For this review, take the finished solid that the model builds, in its own axes (mm). Face numbers are marked on the shaded views. Coordinates: 2 decimals unless noted, no trailing zeros. Loops run counter-clockwise (first coordinate to the right, second up) from the corner with the lowest first, then second, coordinate; pieces in that order, holes last.
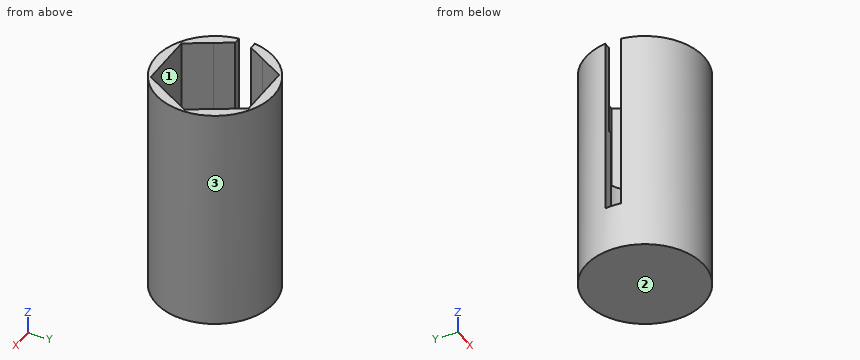
```python
from build123d import *

# Parameters (mm, degrees)
F0_R     = 13
F1_DEPTH = 50
F2_DEPTH = 2
F4_DEPTH = 30
F3_W     = 3.5
F3_H     = 40
F5_DEPTH = 25


with BuildPart() as f1:
    # F0 (on Top) → F1 (new body)
    with BuildSketch(Plane.XY):
        Circle(F0_R)
        Polygon((6.2065153938, 10.75), (9.3097731741, 5.3749998556), (12.4130307876, 0), (9.3097730463, -5.3750000769), (6.2065153938, -10.75), (0, -10.75), (-6.2065153938, -10.75), (-9.3097732188, -5.374999778), (-12.4130307876, 0), (-9.3097730642, 5.3750000458), (-6.2065153938, 10.75), (0, 10.75), align=None, mode=Mode.SUBTRACT)
    extrude(amount=F1_DEPTH)

    # F0 (on Top) → F2 (join)
    with BuildSketch(Plane.XY):
        with BuildLine():
            Line((6.2065153938, -10.75), (9.3097730463, -5.3750000769))
            ThreePointArc((9.3097730463, -5.3750000769), (5.3749999615, -9.3097731129), (0, -10.75))
            Line((0, -10.75), (6.2065153938, -10.75))
        make_face()
        with BuildLine():
            Line((-6.2065153938, -10.75), (0, -10.75))
            ThreePointArc((0, -10.75), (-5.375000111, -9.3097730266), (-9.3097732188, -5.374999778))
            Line((-9.3097732188, -5.374999778), (-6.2065153938, -10.75))
        make_face()
        with BuildLine():
            ThreePointArc((9.3097730463, -5.3750000769), (10.3837026211, -2.7823047777), (10.75, 0))
            ThreePointArc((10.75, 0), (10.3837026542, 2.7823046543), (9.3097731741, 5.3749998556))
            ThreePointArc((9.3097731741, 5.3749998556), (5.3750000722, 9.309773049), (0, 10.75))
            ThreePointArc((0, 10.75), (-5.3749999771, 9.3097731039), (-9.3097730642, 5.3750000458))
            ThreePointArc((-9.3097730642, 5.3750000458), (-10.75, 1.546e-07), (-9.3097732188, -5.374999778))
            ThreePointArc((-9.3097732188, -5.374999778), (-5.375000111, -9.3097730266), (0, -10.75))
            ThreePointArc((0, -10.75), (5.3749999615, -9.3097731129), (9.3097730463, -5.3750000769))
        make_face()
        with BuildLine():
            ThreePointArc((-9.3097730642, 5.3750000458), (-5.3749999771, 9.3097731039), (0, 10.75))
            Line((0, 10.75), (-6.2065153938, 10.75))
            Line((-6.2065153938, 10.75), (-9.3097730642, 5.3750000458))
        make_face()
        with BuildLine():
            ThreePointArc((-9.3097732188, -5.374999778), (-10.75, 1.546e-07), (-9.3097730642, 5.3750000458))
            Line((-9.3097730642, 5.3750000458), (-12.4130307876, 0))
            Line((-12.4130307876, 0), (-9.3097732188, -5.374999778))
        make_face()
        with BuildLine():
            ThreePointArc((0, 10.75), (5.3750000722, 9.309773049), (9.3097731741, 5.3749998556))
            Line((9.3097731741, 5.3749998556), (6.2065153938, 10.75))
            Line((6.2065153938, 10.75), (0, 10.75))
        make_face()
        with BuildLine():
            ThreePointArc((9.3097731741, 5.3749998556), (10.3837026542, 2.7823046543), (10.75, 0))
            ThreePointArc((10.75, 0), (10.3837026211, -2.7823047777), (9.3097730463, -5.3750000769))
            Line((9.3097730463, -5.3750000769), (12.4130307876, 0))
            Line((12.4130307876, 0), (9.3097731741, 5.3749998556))
        make_face()
    extrude(amount=F2_DEPTH)

    # F0 (on Top) → F4 (join)
    with BuildSketch(Plane.XY):
        with BuildLine():
            ThreePointArc((0, 10.75), (5.3750000722, 9.309773049), (9.3097731741, 5.3749998556))
            Line((9.3097731741, 5.3749998556), (6.2065153938, 10.75))
            Line((6.2065153938, 10.75), (0, 10.75))
        make_face()
        with BuildLine():
            ThreePointArc((-9.3097730642, 5.3750000458), (-5.3749999771, 9.3097731039), (0, 10.75))
            Line((0, 10.75), (-6.2065153938, 10.75))
            Line((-6.2065153938, 10.75), (-9.3097730642, 5.3750000458))
        make_face()
        with BuildLine():
            ThreePointArc((-9.3097732188, -5.374999778), (-10.75, 1.546e-07), (-9.3097730642, 5.3750000458))
            Line((-9.3097730642, 5.3750000458), (-12.4130307876, 0))
            Line((-12.4130307876, 0), (-9.3097732188, -5.374999778))
        make_face()
        with BuildLine():
            Line((-6.2065153938, -10.75), (0, -10.75))
            ThreePointArc((0, -10.75), (-5.375000111, -9.3097730266), (-9.3097732188, -5.374999778))
            Line((-9.3097732188, -5.374999778), (-6.2065153938, -10.75))
        make_face()
        with BuildLine():
            Line((6.2065153938, -10.75), (9.3097730463, -5.3750000769))
            ThreePointArc((9.3097730463, -5.3750000769), (5.3749999615, -9.3097731129), (0, -10.75))
            Line((0, -10.75), (6.2065153938, -10.75))
        make_face()
        with BuildLine():
            ThreePointArc((9.3097731741, 5.3749998556), (10.3837026542, 2.7823046543), (10.75, 0))
            ThreePointArc((10.75, 0), (10.3837026211, -2.7823047777), (9.3097730463, -5.3750000769))
            Line((9.3097730463, -5.3750000769), (12.4130307876, 0))
            Line((12.4130307876, 0), (9.3097731741, 5.3749998556))
        make_face()
    extrude(amount=F4_DEPTH)

    # F3 (on Right) → F5 (cut)
    with BuildSketch(Plane.YZ):
        with Locations((0.0118296053, 30.4367649183)):
            Rectangle(F3_W, F3_H)
    extrude(amount=-F5_DEPTH, mode=Mode.SUBTRACT)


solid = f1.part
```
Q1. The part is to be moulded in two halves that separate along Y. For the marked faces 1, 2 and 3, say which applies: +Y half, -Y half, draft (parallel to the pull), parting line (faces both ways), or undercut.
Q2. Consider section A-A (z = 5). State the section outline as (x, y) points, then the cut area to 3 significant figures.
Q3. Consider section D-D (z = 27). State the section outline as (x, y) points.
Q4. Consider section B-B (x = 3.75). State the section outline as (y, z) points.
Q5. Wall thickness on probe 1 along Y at (x, z) = (0, 15); probe 2 along Z at (x, y) = (8, 3.25); probe 3 along X at (y, z) = (0, 17): over which ranges is each line inside the solid? List them lowest first.
Q6. For pin 1 Ø1 at (x, z) = (2, 32) entering from +Y; pin 2 Ø5 at (y, z) = (-3.5, 5.5) entering from +X; pin 3 Ø6 at (y, z) = (-7, 45) entering from -X; pin 4 Ø3.5 at (x, z) = (1, 42) entering from +Y, all flat-tipped, find the tip position at first contact; note any pin that passes through.
Model answer:
1. face 1: undercut
1. face 2: draft
1. face 3: parting line
2. outline: circle Ø26 at (0, 0); hole circle Ø21.5 at (0, 0)
2. area: 168 mm2
3. outline: (-12.88, -1.74) arc R13 ccw (long way) to (-12.88, 1.76) - (-10.6, 1.76) arc R10.75 cw (long way) to (-10.61, -1.74) - close
4. outline: (-12.45, 0) - (12.45, 0) - (12.45, 50) - (10.75, 50) - (10.75, 30) - (10.07, 30) - (10.07, 2) - (-10.07, 2) - (-10.07, 30) - (-10.75, 30) - (-10.75, 50) - (-12.45, 50) - close
5. probe 1: y = -13 to -10.75, 10.75 to 13
5. probe 2: z = 0 to 2
5. probe 3: x = 10.75 to 13
6. pin 1: stops at y = 12.91
6. pin 2: stops at x = 12.96
6. pin 3: stops at x = -12.37
6. pin 4: stops at y = 13
